Geometry check sheet. Reference: drawing and pictorial views, mm from the part's lowest x, y, z. A direction names the side the tool comes from. Round coordinates to 2 decimals unless told otherwise and drop trailing zeros. Order: outer loops, then holes, each group sorted by start corner. A loop starts at its lowest first (then second) coordinate and runs counter-clockwise, first axis right, second up.
(1) Sectioned sample at C-C (z = 9.5). Record the boundary of the cut face in (x, y) (1 decimal).
(2) Sectioned sample at B-B (x = 29.5). Record the boundary of the cut face in (y, z) (1 decimal).
(3) Go/stop test with flat-tipped pins: pin 1 (1.5 mm diameter, centred on y = 7.5, z = 16.5, fed in from +X); pin 2 (2 mm diameter, centred on x = 1, y = 10, fed in from -Z); pin 3 (1.2 mm diameter, centred on x = 6, z = 17, fed in from -Y). Record where each tip stops, or that it passes through.
(4) Material ranges on line 1 along X through (y, z) = (1.75, 11); line 2 along Z through (x, y) = (6.5, 13.75); line 3 along X through (y, z) = (8.5, 17.75), recorded low to high.
(5) Set-up check for the marked faces 1, 2 and 3: record each of +Z, -Z, +X, -X, +Y, -Y from which the full face is reachable in a straight line by a thin tool's end or side.
(6) Sectioned sample at A-A (y = 10.75). Record the boundary of the cut face in (x, z) (1 decimal), plus the area to 3 significant figures.
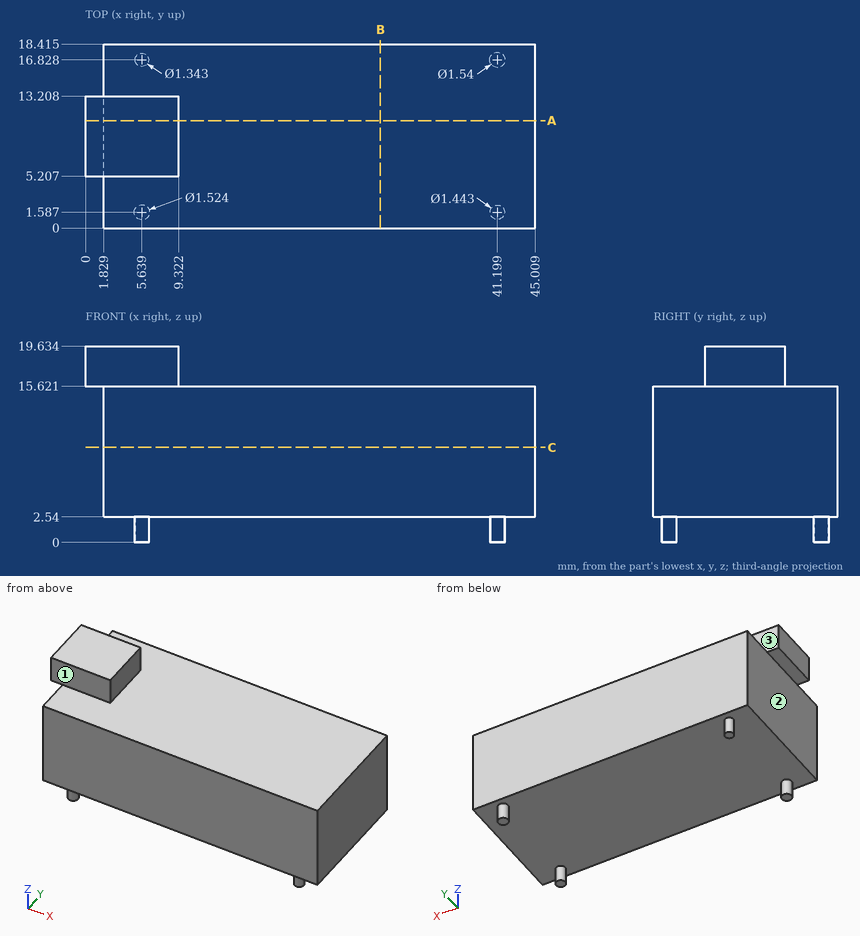
Answer below:
1. outline: (1.8, 0) - (45, 0) - (45, 18.4) - (1.8, 18.4) - close
2. outline: (0, 2.5) - (18.4, 2.5) - (18.4, 15.6) - (0, 15.6) - close
3. pin 1: stops at x = 9.32
3. pin 2: stops at z = 2.54
3. pin 3: stops at y = 5.21
4. line 1: x = 1.83 to 45.01
4. line 2: z = 2.54 to 15.62
4. line 3: x = 0 to 9.32
5. face 1: +Z, +X, -X, -Y
5. face 2: -Z, -X, +Y, -Y
5. face 3: +Z, +X, -X, +Y
6. outline: (0, 15.6) - (1.8, 15.6) - (1.8, 2.5) - (45, 2.5) - (45, 15.6) - (9.3, 15.6) - (9.3, 19.6) - (0, 19.6) - close
6. area: 602 mm2
